from build123d import *

# Parameters (mm, degrees)
SKETCH_1_R               = 139
SKETCH_1_R_2             = 61
EXTRUDE_1_DEPTH          = 10
CUT_EXTRUDE_1_DEPTH      = 5
PATTERN_CIRCULAR_2_COUNT = 14
SKETCH_3_R               = 5.1
CUT_EXTRUDE_2_DEPTH      = 197.829875781
SKETCH_8_R               = 5.1
CUT_EXTRUDE_3_DEPTH      = 197.829875781
SKETCH_10_R              = 2.5
CUT_EXTRUDE_4_DEPTH      = 197.829875781
MIRROR_2_COPY_1_SKETCH_R = 5.1
MIRROR_2_COPY_1_DEPTH    = 197.829875781
M5_BASE_PLATE_D          = 5.8


with BuildPart() as part:
    # ｽｹｯﾁ1 → ﾎﾞｽ - 押し出し1 (new body)
    with BuildSketch(Plane(origin=(0, 0, 0), x_dir=(1, 0, 0), z_dir=(0, 1, 0))):
        with Locations(Location((0, 0, 0), (0, 0, 270))):
            Circle(SKETCH_1_R)
        with Locations(Location((0, 0, 0), (0, 0, 270))):
            Circle(SKETCH_1_R_2, mode=Mode.SUBTRACT)
    extrude(amount=EXTRUDE_1_DEPTH)

    # ｽｹｯﾁ2 → ｶｯﾄ - 押し出し1 (cut)
    with BuildSketch(Plane(origin=(0, 10, 0), x_dir=(1, 0, 0), z_dir=(0, 1, 0))):
        with BuildLine():
            Line((18.5, 119), (18.5, 85))
            ThreePointArc((18.5, 85), (0, 66.5), (-18.5, 85))
            Line((-18.5, 85), (-18.5, 119))
            ThreePointArc((-18.5, 119), (0, 137.5), (18.5, 119))
        make_face()
    cut_extrude_1 = extrude(amount=-CUT_EXTRUDE_1_DEPTH, mode=Mode.SUBTRACT)

    # 円形ﾊﾟﾀｰﾝ2: ｶｯﾄ - 押し出し1 ×14 about axis
    pattern_circular_2_axis = Axis((0, 0, 0), (0, 1, 0))
    for i in range(1, PATTERN_CIRCULAR_2_COUNT):
        add(cut_extrude_1.rotate(pattern_circular_2_axis, i * 360 / PATTERN_CIRCULAR_2_COUNT), mode=Mode.SUBTRACT)

    # ｽｹｯﾁ3 → ｶｯﾄ - 押し出し2 (cut, through all)
    with BuildSketch(Plane(origin=(0, 10, 0), x_dir=(1, 0, 0), z_dir=(0, 1, 0))):
        with Locations(Location((130, 0, 0), (0, 0, 270))):
            Circle(SKETCH_3_R)
    cut_extrude_2 = extrude(amount=-CUT_EXTRUDE_2_DEPTH, mode=Mode.SUBTRACT)

    # ｽｹｯﾁ8 → ｶｯﾄ - 押し出し3 (cut, through all)
    with BuildSketch(Plane(origin=(0, 10, 0), x_dir=(1, 0, 0), z_dir=(0, 1, 0))):
        with Locations(Location((81.053674242, 101.638092721, 0), (0, 0, 270))):
            Circle(SKETCH_8_R)
    cut_extrude_3 = extrude(amount=-CUT_EXTRUDE_3_DEPTH, mode=Mode.SUBTRACT)

    # ｽｹｯﾁ10 → ｶｯﾄ - 押し出し4 (cut, through all)
    with BuildSketch(Plane(origin=(0, 10, 0), x_dir=(1, 0, 0), z_dir=(0, 1, 0))):
        with Locations((-139, 0)):
            Circle(SKETCH_10_R)
    extrude(amount=-CUT_EXTRUDE_4_DEPTH, mode=Mode.SUBTRACT)

    # ﾐﾗｰ1: ｶｯﾄ - 押し出し3 across plane
    add(cut_extrude_3.mirror(Plane.XY), mode=Mode.SUBTRACT)

    # ﾐﾗｰ2: ｶｯﾄ - 押し出し2, ｶｯﾄ - 押し出し3 across plane
    add(cut_extrude_2.mirror(Plane(origin=(0, 0, 0), x_dir=(0, 0, 1), z_dir=(1, 0, 0))), mode=Mode.SUBTRACT)
    add(cut_extrude_3.mirror(Plane(origin=(0, 0, 0), x_dir=(0, 0, 1), z_dir=(1, 0, 0))), mode=Mode.SUBTRACT)

    # ﾐﾗｰ2 copy 1 sketch → ﾐﾗｰ2 copy 1 (cut, through all)
    with BuildSketch(Plane(origin=(0, 10, 0), x_dir=(-1, 0, 0), z_dir=(0, 1, 0))):
        with Locations(Location((81.053674242, 101.638092721, 0), (0, 0, 270))):
            Circle(MIRROR_2_COPY_1_SKETCH_R)
    extrude(amount=-MIRROR_2_COPY_1_DEPTH, mode=Mode.SUBTRACT)

    # M5 Base_Plateへの固定用穴 (through all)
    with Locations(Plane(origin=(71.701327214, 10, -89.910620484), x_dir=(0, 0, 1), z_dir=(0, 1, 0))):
        with Locations((0, 0), (89.910620484, 43.298672786), (179.821240968, 0), (179.821240968, -143.402654428), (89.910620484, -186.701327214), (0, -143.402654428)):
            Hole(M5_BASE_PLATE_D / 2)


solid = part.part
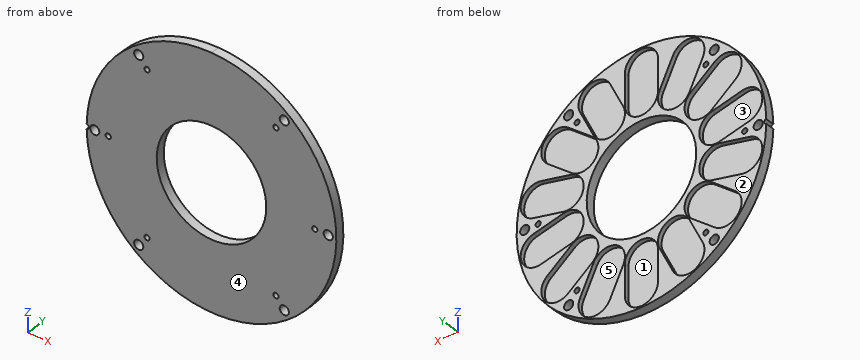
Design review of the part built by this model. Coordinates are the model's own, in mm. Face numbers are marked on the shaded views. A direction names the side the tool comes from. Round coordinates to 2 decimals unless told otherwise and drop trailing zeros. Order: outer loops, then holes, each group sorted by start corner. A loop starts at its lowest first (then second) coordinate and runs counter-clockwise, first axis right, second up. Notation, with made-up numbers: M 30,66.5 L 58,66.5 A18 ccw 58,79.5 Z; hole C 47,69 d8. An arc over 180 degrees is marked long. Answer as CSV lines item,"result". Start each with the question number.
1) Add section A-A (x = -130). Give the boundary of the cut face in (y, z).
2) For pin 1 Ø5 at (x, z) = (33.5, 93.5) entering from +Y; pin 2 Ø9 at (x, z) = (81.05, 101.64) entering from -Y; pin 3 Ø1.5 at (x, y) = (78.5, 3) entering from -Z; pin 4 Ø10 at (x, z) = (-13, -75) entering from -Y, all flat-tipped, find the tip position at first contact; note any pin that passes through.
3) The part is to be moulded in two halves that separate along X. For the marked faces 1, 2 and 3, say which applies: +X half, -X half, draft (parallel to the pull), parting line (faces both ways), or undercut.
4) Tool access review of the marked faces 4 and 5: name each direction out of +Z, -Z, +X, -X, +Y, -Y from which nothing blocks a thin tool from reaching the whole face with its end or side.
5) Wall thickness on line 1 along X through (y, z) = (5.5, 0); line 2 along X through (y, z) = (7.5, -77.5); line 3 along Z through (x, y) = (-24, 8.25): over which ranges is each line inside the solid? List them lowest first. Write a range as [from, to].
6) Add section C-C (y = 8). Give the number of separate pieces and of enclosed holes in the cut face, then the cut area to 3 significant figures.
7) Add section B-B (z = -14). Give the boundary of the cut face in (x, y), then the cut area to 3 significant figures.
Resolved:
1,outline,"M 0,-49.2 L 10,-49.2 L 10,-38.59 L 5,-38.59 L 5,-14.37 L 10,-14.37 L 10,-5.1 L 0,-5.1 Z; M 0,5.1 L 10,5.1 L 10,14.37 L 5,14.37 L 5,38.59 L 10,38.59 L 10,49.2 L 0,49.2 Z"
2,pin 1,"y = 5"
2,pin 2,"through"
2,pin 3,"z = -115.22"
2,pin 4,"y = 0"
3,face 1,"undercut"
3,face 2,"draft"
3,face 3,"undercut"
4,face 4,"+Z, -Z, +X, -X, -Y"
4,face 5,"+Y"
5,line 1,"[-136.5, -135.1], [-124.9, -117.9], [-112.1, -61], [61, 112.1], [117.9, 124.9], [135.1, 139]"
5,line 2,"[-115.39, -111.24], [-67.51, -57.86], [-18.4, -16.91], [16.91, 18.4], [57.86, 67.51], [111.24, 115.39]"
5,line 3,"[-136.91, -92.47], [-63.3, -56.08], [56.08, 63.3], [92.47, 136.91]"
6,separate pieces,"1"
6,enclosed holes,"27"
6,area,"15,700 mm^2"
7,outline,"M -138.29,0 L -59.37,0 L -59.37,10 L -65.03,10 L -65.03,5 L -129.67,5 L -129.67,10 L -138.29,10 Z; M 59.37,0 L 138.29,0 L 138.29,10 L 129.67,10 L 129.67,5 L 65.03,5 L 65.03,10 L 59.37,10 Z"
7,area,"932 mm^2"
